Could you check a few things on this model? Use its own coordinates, in mm. Give positions to 0.01 mm unless a question says otherwise; leave off trailing zeros. Loops run counter-clockwise (first coordinate to the right, second up) from the corner with the lowest first, then second, coordinate; pieces in that order, holes last. Notation, with made-up numbers: M -8.75,-7 L 15.25,-7 A35 ccw 15.25,27 Z; hole C 26.5,-40 d11. An arc over 180 degrees is marked long. Return JSON: item names as keys, results as strings. Group by question number.
1. Please list where these lines run through material, in increasing order: line 1 (X direction, y = 2.2, z = -2); line 2 (X direction, y = 2.5, z = 7); line 3 (Z direction, x = -11.5, y = 0.7).
2. If we section it at D-D (x = -38): Write out the boundary of the cut face in (y, z).
3. If we section it at B-B (z = 13): Write out the boundary of the cut face in (x, y).
4. If we section it at A-A (x = 0): Write out the boundary of the cut face in (y, z).
5. If we section it at C-C (y = 3.75): Write out the boundary of the cut face in (x, z).
6. For pin 1 (2.5 mm diameter, centred on x = 30, y = 1.5, fed in from +Z); pin 2 (2.5 mm diameter, centred on y = 3.5, z = 0.5, fed in from +X); pin 3 (2.5 mm diameter, centred on y = 2, z = 1, fed in from -X), each with a flat end and sliding along its axis, tell me the tip position at first contact or that it passes through.
```python
from build123d import *

# Parameters (mm, degrees)
SKETCH1_R           = 49.95
SKETCH1_R_2         = 1
BOSS_EXTRUDE1_DEPTH = 4.75


with BuildPart() as part:
    # Sketch1 → Boss-Extrude1 (new body)
    with BuildSketch(Plane(origin=(0, 0, 0), x_dir=(1, 0, 0), z_dir=(0, 1, 0))):
        with Locations(Location((0, 0, 0), (0, 0, 270))):
            Circle(SKETCH1_R)
        with Locations(Location((-28.698085879, -2, 0), (0, 0, 270))):
            Circle(SKETCH1_R_2, mode=Mode.SUBTRACT)
        with Locations(Location((-28.698085879, 2, 0), (0, 0, 90))):
            Circle(SKETCH1_R_2, mode=Mode.SUBTRACT)
        with Locations(Location((28.698085879, -2, 0), (0, 0, 90))):
            Circle(SKETCH1_R_2, mode=Mode.SUBTRACT)
        with Locations(Location((28.698085879, 2, 0), (0, 0, 270))):
            Circle(SKETCH1_R_2, mode=Mode.SUBTRACT)
        with BuildLine():
            Line((-32.306829346, -5), (-26.698085879, -5))
            ThreePointArc((-26.698085879, -5), (-25.283872317, -4.414213562), (-24.698085879, -3))
            Line((-24.698085879, -3), (-24.698085879, 3))
            ThreePointArc((-24.698085879, 3), (-25.283872317, 4.414213562), (-26.698085879, 5))
            Line((-26.698085879, 5), (-32.306829346, 5))
            ThreePointArc((-32.306829346, 5), (-33.863594421, 5.744419457), (-34.261473284, 7.423517499))
            ThreePointArc((-34.261473284, 7.423517499), (0, 35.05648533), (34.261473284, 7.423517499))
            ThreePointArc((34.261473284, 7.423517499), (33.863594421, 5.744419457), (32.306829346, 5))
            Line((32.306829346, 5), (26.698085879, 5))
            ThreePointArc((26.698085879, 5), (25.283872317, 4.414213562), (24.698085879, 3))
            Line((24.698085879, 3), (24.698085879, -3))
            ThreePointArc((24.698085879, -3), (25.283872317, -4.414213562), (26.698085879, -5))
            Line((26.698085879, -5), (32.306829346, -5))
            ThreePointArc((32.306829346, -5), (33.863594421, -5.744419457), (34.261473284, -7.423517499))
            ThreePointArc((34.261473284, -7.423517499), (0, -35.05648533), (-34.261473284, -7.423517499))
            ThreePointArc((-34.261473284, -7.423517499), (-33.863594421, -5.744419457), (-32.306829346, -5))
        make_face(mode=Mode.SUBTRACT)
    extrude(amount=BOSS_EXTRUDE1_DEPTH)


solid = part.part
```
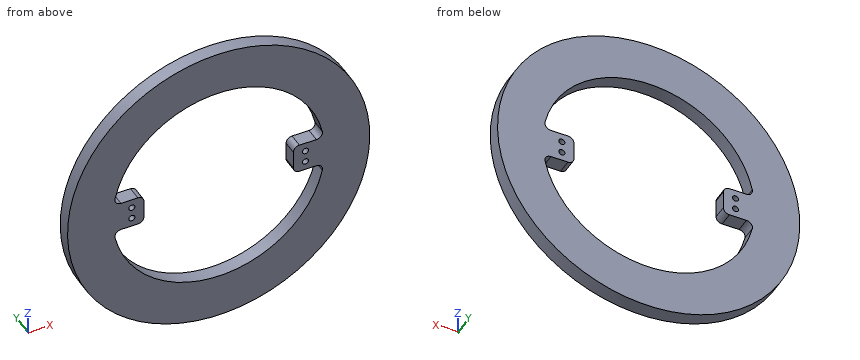
Answer:
{
 "1": {"line 1": "x = -49.91 to -29.7, -27.7 to -24.7, 24.7 to 27.7, 29.7 to 49.91", "line 2": "x = -49.46 to -34.31, 34.31 to 49.46", "line 3": "z = -48.61 to -33.12, 33.12 to 48.61"},
 "2": {"outline": "M 0,-32.42 L 4.75,-32.42 L 4.75,32.42 L 0,32.42 Z"},
 "3": {"outline": "M -48.23,0 L -32.56,0 L -32.56,4.75 L -48.23,4.75 Z; M 32.56,0 L 48.23,0 L 48.23,4.75 L 32.56,4.75 Z"},
 "4": {"outline": "M 0,-49.95 L 4.75,-49.95 L 4.75,-35.06 L 0,-35.06 Z; M 0,35.06 L 4.75,35.06 L 4.75,49.95 L 0,49.95 Z"},
 "5": {"outline": "C 0,0 d99.9; hole M -34.26,-7.42 A35.06 ccw 34.26,-7.42 A2 ccw 32.31,-5 L 26.7,-5 A2 cw 24.7,-3 L 24.7,3 A2 cw 26.7,5 L 32.31,5 A2 ccw 34.26,7.42 A35.06 ccw -34.26,7.42 A2 ccw -32.31,5 L -26.7,5 A2 cw -24.7,3 L -24.7,-3 A2 cw -26.7,-5 L -32.31,-5 A2 ccw Z; hole C -28.7,-2 d2; hole C -28.7,2 d2; hole C 28.7,-2 d2; hole C 28.7,2 d2"},
 "6": {"pin 1": "stops at z = 40.85", "pin 2": "stops at x = 49.95", "pin 3": "stops at x = -49.95"}
}
